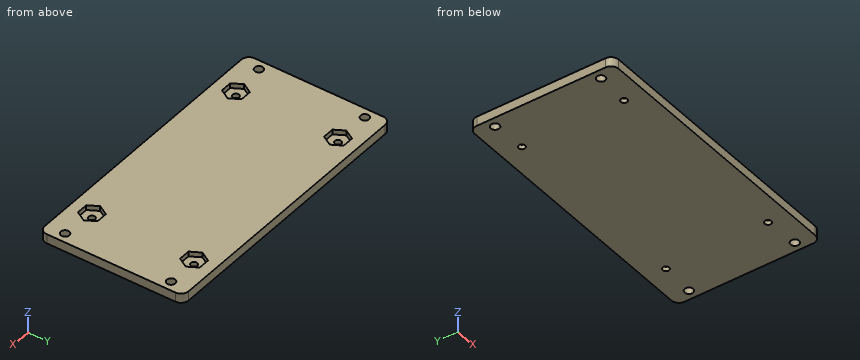
```python
from build123d import *

# Parameters (mm, degrees)
SKETCH1_W               = 150
SKETCH1_H               = 76
BOSS_EXTRUDE1_DEPTH     = 5
FILLET1_R               = 4
SKETCH2_R               = 1.7
CUT_EXTRUDE1_DEPTH      = 85.225886757
CUT_EXTRUDE2_DEPTH      = 2.6
CUT_EXTRUDE3_DEPTH      = 85.225886757
CUT_EXTRUDE3_DEPTH_BACK = 85.225886757
SKETCH4_R               = 2.25


with BuildPart() as part:
    # Sketch1 → Boss-Extrude1 (new body)
    with BuildSketch(Plane.XY):
        Rectangle(SKETCH1_W, SKETCH1_H)
    extrude(amount=BOSS_EXTRUDE1_DEPTH)

    # Fillet1
    fillet1_edges = [part.edges().sort_by_distance(p)[0] for p in [
        (-75, 38, 2.5),
        (75, 38, 2.5),
        (75, -38, 2.5),
        (-75, -38, 2.5),
    ]]
    fillet(fillet1_edges, radius=FILLET1_R)

    # Sketch2 → Cut-Extrude1 (cut, through all)
    with BuildSketch(Plane(origin=(0, 0, 0), x_dir=(-1, 0, 0), z_dir=(0, 0, -1))):
        with Locations((52, -27)):
            Circle(SKETCH2_R)
        with Locations(Location((52, 27, 0), (0, 0, 180))):
            Circle(SKETCH2_R)
        with Locations((-52, 27)):
            Circle(SKETCH2_R)
        with Locations(Location((-52, -27, 0), (0, 0, 180))):
            Circle(SKETCH2_R)
    extrude(amount=-CUT_EXTRUDE1_DEPTH, mode=Mode.SUBTRACT)

    # Sketch3 → Cut-Extrude2 (cut)
    with BuildSketch(Plane.XY.offset(5)):
        Polygon((-49, 21.803847577), (-46, 27), (-49, 32.196152423), (-55, 32.196152423), (-58, 27), (-55, 21.803847577), align=None)
        Polygon((55, 21.803847577), (49, 21.803847577), (46, 27), (49, 32.196152423), (55, 32.196152423), (58, 27), align=None)
        Polygon((49, -21.803847577), (46, -27), (49, -32.196152423), (55, -32.196152423), (58, -27), (55, -21.803847577), align=None)
        Polygon((-55, -21.803847577), (-49, -21.803847577), (-46, -27), (-49, -32.196152423), (-55, -32.196152423), (-58, -27), align=None)
    extrude(amount=-CUT_EXTRUDE2_DEPTH, mode=Mode.SUBTRACT)

    # Sketch4 → Cut-Extrude3 (cut, two sides: drawn at the far end of the back side and taken through both)
    with BuildSketch(Plane.XY.offset(5).offset(-CUT_EXTRUDE3_DEPTH_BACK)):
        with Locations((-70, 28)):
            Circle(SKETCH4_R)
        with Locations((70, 28)):
            Circle(SKETCH4_R)
        with Locations((70, -28)):
            Circle(SKETCH4_R)
        with Locations((-70, -28)):
            Circle(SKETCH4_R)
    extrude(amount=CUT_EXTRUDE3_DEPTH + CUT_EXTRUDE3_DEPTH_BACK, mode=Mode.SUBTRACT)


solid = part.part
```
Could you check a few things on this model? Use its own coordinates, in mm. Round coordinates to 2 decimals unless told otherwise and drop trailing zeros. Write each loop counter-clockwise with the first axis right and the second up, starting at its lowest first coordinate (ties: lowest second). Pieces come first, ordered by that corner, then holes. Notation, with made-up numbers: M 33,28 L 60,28 A36 cw 60,67 Z; hole C 1.25,35 d9. An arc over 180 degrees is marked long. Answer in a Markdown table with one row per item. Add a question column.
Q1. Imagine slicing it at B-B (z = 3.2). Give the number of separate pieces and of enclosed holes in the cut face, then the cut area to 3 significant figures.
Q2. If I drill on line 1 (Y direction, x = -52, z = 1.75); line 2 (X direction, y = 23, z = 4.1); line 3 (X direction, y = -22, z = 3.75), over which ranges is the centre line in solid material (lowest first)? Write a range as from..to.
Q3. Imagine slicing it at A-A (x = 52). Please give me the cut outline in (y, z), then the cut area to 3 significant figures.
Q4. Will this pin go through, and if not, where does the flat tip stop? pin 1 Ø3 at (x, y) = (-52, 24.5) entering from +Z.
Values:
| question | item | result |
|---|---|---|
| 1 | separate pieces | 1 |
| 1 | enclosed holes | 8 |
| 1 | area | 10,900 mm^2 |
| 2 | line 1 | -38..-28.7, -25.3..25.3, 28.7..38 |
| 2 | line 2 | -75..-55.69, -48.31..48.31, 55.69..75 |
| 2 | line 3 | -75..-55.11, -48.89..48.89, 55.11..75 |
| 3 | outline | M -38,0 L -28.7,0 L -28.7,2.4 L -32.2,2.4 L -32.2,5 L -38,5 Z; M -25.3,0 L 25.3,0 L 25.3,2.4 L 21.8,2.4 L 21.8,5 L -21.8,5 L -21.8,2.4 L -25.3,2.4 Z; M 28.7,0 L 38,0 L 38,5 L 32.2,5 L 32.2,2.4 L 28.7,2.4 Z |
| 3 | area | 310 mm^2 |
| 4 | pin 1 | z = 2.4 |
